Build history of the part. All positions in model axes, mm. A direction names the side the tool comes from. Round coordinates to 2 decimals unless told otherwise and drop trailing zeros. Loops run counter-clockwise (first coordinate to the right, second up) from the corner with the lowest first, then second, coordinate; pieces in that order, holes last. Notation, with made-up numbers: (9.5, 78.25) -> (27.5, 78.25) arc R23 cw to (27.5, 106.25) -> close; hole circle Ø1 at (-33, 7.5). An arc over 180 degrees is marked (long way). Put each result on its own line as item: value. Start each with the question number.
Autodesk Inventor part; units mm, degrees
ref_plane "YZ Plane" through (0, 0, 0) normal (1, 0, 0) x (0, 1, 0)
ref_plane "XZ Plane" through (0, 0, 0) normal (0, 1, 0) x (-1, 0, 0)
ref_plane "XY Plane" through (0, 0, 0) normal (0, 0, 1) x (1, 0, 0)
sketch "Skizze1" plane through (0, 0, 0) normal (0, 0, 1) x (1, 0, 0)
  line L0 (0, 80) -> (24, 80)
  line L1 (24, 80) -> (24, -80)
  line L2 (24, -80) -> (0, -80)
  line L3 (0, -80) -> (0, 80)
  line L4 (24, 40) -> (124, 40)
  line L5 (124, 40) -> (124, -40)
  line L6 (124, -40) -> (24, -40)
  line L7 (24, -40) -> (24, 40)
  point P0 (0, 0)
  point P1 (24, 0)
  point P2 (0, 0)
  point P3 (94, 0)
  point P4 (124, 0)
  dimension "d0" = 160
  dimension "d1" = 24
  dimension "d2" = 124
  dimension "d3" = 80
  dimension "d4" = 94
extrude "Extrusion1" add sketch "Skizze1" along normal mid plane 160 contours L0 L1 L2 L3
sketch "Skizze2" plane through (24, -80, 80) normal (1, 0, 0) x (0, 0, -1)
  line L0 (0, 160) -> (30, 160)
  line L1 (30, 160) -> (30, 130)
  line L2 (30, 130) -> (0, 130)
  line L3 (0, 130) -> (0, 160)
  point P0 (80, 80)
  dimension "d19" = 30
  dimension "d20" = 30
extrude "Extrusion4" cut sketch "Skizze2" against normal blind 9
pattern_circular "Runde Anordnung1" count 4 over 360 about axis through (-10, 0, 0) along (1, 0, 0) of "Extrusion4"
sketch "Skizze3" plane through (24, 50, 50) normal (1, 0, 0) x (0, 0, -1)
  line L0 (-15, 15) -> (115, 15)
  line L1 (115, 15) -> (115, -115)
  line L2 (115, -115) -> (-15, -115)
  line L3 (-15, -115) -> (-15, 15)
  line L4 (-15, 15) -> (115, -115) construction
  line L5 (115, 15) -> (-15, -115) construction
  point P0 (50, -50)
  dimension "d26" = 130
  dimension "d27" = 130
hole "Bohrung2" at (24, 65, 65) at (24, -65, 65) at (24, 65, -65) at (24, -65, -65) direction (-1, 0, 0) diameter 10.5 end through all
fillet "Rundung2" radius 15 4 edges at (7.5, 80, -80) (7.5, -80, -80) (7.5, -80, 80) (7.5, 80, 80)
fillet "Rundung3" radius 10 4 edges at (19.5, -50, 50) (19.5, -50, -50) (19.5, 50, -50) (19.5, 50, 50)
equation "\"d5\" = d0"
properties part number "Gelenkflansch_Hinten_ohne_halterung" material "Stahl AISI 4130"
Item 1: Wall check: line 1 (Y direction, x = 6.5, z = 65); line 2 (X direction, y = 67.5, z = 52.5). Give the ranges that are in metal, low to high. Write a range as from..to.
Item 2: Drop flat-ended pins along their axis: pin 1 (24 mm diameter, centred on y = 61, z = 71.5, fed in from +X); pin 2 (10 mm diameter, centred on x = 19, y = 72, fed in from -Z); pin 3 (10 mm diameter, centred on x = 20.5, z = 68, fed in from -Y); pin 4 (2.5 mm diameter, centred on x = 21.5, y = -72.5, fed in from -Z). Give the stop position or say it passes through.
Item 3: Pull direction Y, two halves, no side cores. Call faces 1 (the face through (15, -59, 65)), 2 (the face through (7.4, 68.19, -60.83)), 3 (the face through (19.44, 53.01, 52.85)): +Y half, -Y half, draft (parallel to the pull), parting line (faces both ways), or undercut.
Item 4: 3-axis set-ups, long thin cutter, end or side, ignore diameter. For faces 4 (the face through (7.4, -75.72, 75.49)), 5 (the face through (19.44, 52.85, -53.01)), 6 (the face through (20, 70, 50)), 7 (the face through (19.44, -53.01, -52.85)), 8 (the face through (20, -70, 50)): which of +Z, -Z, +X, -X, +Y, -Y reach the whole face in a straight line?
Item 5: Cut at B-B on z = 67. Write the cut outline in (x, y).
Item 6: Cut at C-C on z = -55. Write the cut outline in (x, y).
Item 7: Cut at A-A on x = 20. Write the cut outline in (y, z), then the cut area to 3 significant figures.
Ans:
1. line 1: y = -80..-70.25, -59.75..59.75, 70.25..80
1. line 2: x = 0..15
2. pin 1: stops at x = 24
2. pin 2: stops at z = -79.46
2. pin 3: stops at y = -50
2. pin 4: stops at z = -50
3. face 1: draft
3. face 2: undercut
3. face 3: +Y half
4. face 4: +Z, +X, -X, -Y
4. face 5: -Z, +X, +Y
4. face 6: +Z, +X, +Y
4. face 7: -Z, +X, -Y
4. face 8: +Z, +X, -Y
5. outline: (0, -79.87) -> (15, -79.87) -> (15, -69.85) -> (0, -69.85) -> close; (0, -60.15) -> (15, -60.15) -> (15, -50) -> (24, -50) -> (24, 50) -> (15, 50) -> (15, 60.15) -> (0, 60.15) -> close; (0, 69.85) -> (15, 69.85) -> (15, 79.87) -> (0, 79.87) -> close
6. outline: (0, -80) -> (15, -80) -> (15, -51.34) -> (24, -51.34) -> (24, 51.34) -> (15, 51.34) -> (15, 80) -> (0, 80) -> close
7. outline: (-80, -50) -> (-60, -50) arc R10 cw to (-50, -60) -> (-50, -80) -> (50, -80) -> (50, -60) arc R10 cw to (60, -50) -> (80, -50) -> (80, 50) -> (60, 50) arc R10 cw to (50, 60) -> (50, 80) -> (-50, 80) -> (-50, 60) arc R10 cw to (-60, 50) -> (-80, 50) -> close
7. area: 22,100 mm2
